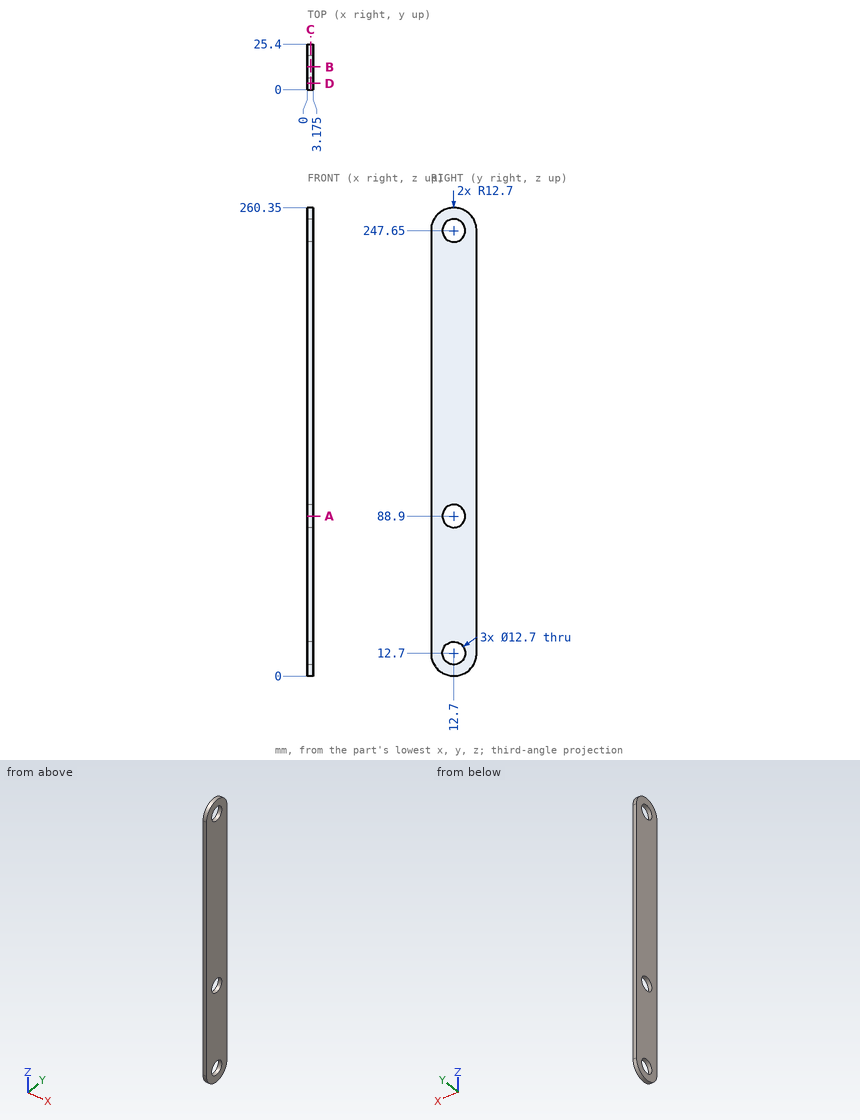
Design review of the part shown in the three views and the two pictorial views. Dimensions are in mm from the part's minimum x, y and z. Give positions to 0.01 mm unless a question says otherwise; leave off trailing zeros. Write each loop counter-clockwise with the first axis right and the second up, starting at its lowest first coordinate (ties: lowest second). Pieces come first, ordered by that corner, then holes. Notation, with made-up numbers: M 75.25,-32 L 109.25,-32 A23 cw 109.25,-4 Z; hole C -29,-35 d11. An arc over 180 degrees is marked long. One line per item, written item: value.
1) Take a section at B-B, the plane y = 12.7. Write out the cut boundary in (x, z) (3 decimals).
Results are:
outline: M 0,0 L 3.175,0 L 3.175,6.35 L 0,6.35 Z; M 0,19.05 L 3.175,19.05 L 3.175,82.55 L 0,82.55 Z; M 0,95.25 L 3.175,95.25 L 3.175,241.3 L 0,241.3 Z; M 0,254 L 3.175,254 L 3.175,260.35 L 0,260.35 Z
2) Take a section at D-D, the plane y = 3.5. Write out the cut boundary in (x, z) (3 decimals), then the cut area to 3 significant figures.
Results are:
outline: M 0,3.945 L 3.175,3.945 L 3.175,256.405 L 0,256.405 Z
area: 802 mm²
3) Take a section at C-C, the plane x = 1.85. Write out the cut boundary in (y, z).
Results are:
outline: M 0,12.7 A12.7 ccw 25.4,12.7 L 25.4,247.65 A12.7 ccw 0,247.65 Z; hole C 12.7,12.7 d12.7; hole C 12.7,88.9 d12.7; hole C 12.7,247.65 d12.7
4) For line 1 (Z direction, x = 1.1, y = 12.7); line 2 (Z direction, x = 1.2, y = 10.75); line 3 (Y direction, x = 1.1, z = 244), list the stretches that pass through material, from the lowest coordinate up. Write a range as from..to.
Results are:
line 1: z = 0..6.35, 19.05..82.55, 95.25..241.3, 254..260.35
line 2: z = 0.15..6.66, 18.74..82.86, 94.94..241.61, 253.69..260.2
line 3: y = 0..7.5, 17.9..25.4
5) For P1, Ø11.5, axis at y = 12.7, z = 12.7, coming from the +X side, flat-tipped, find the tip position at first contact; note if it passes through.
Results are:
P1: passes through
6) Take a section at A-A, the plane z = 88.9. Write out the cut boundary in (x, y) (3 decimals), then the cut area to 3 significant figures.
Results are:
outline: M 0,0 L 3.175,0 L 3.175,6.35 L 0,6.35 Z; M 0,19.05 L 3.175,19.05 L 3.175,25.4 L 0,25.4 Z
area: 40.3 mm²
